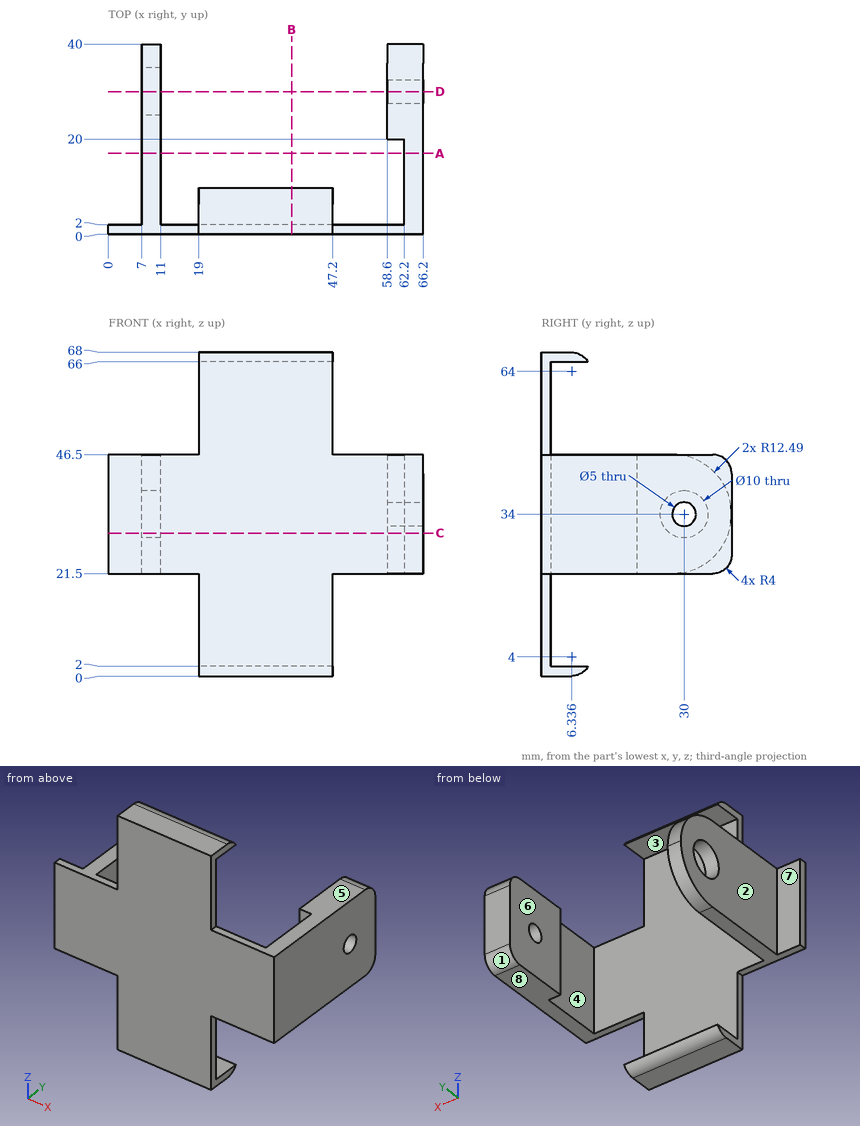
Source: three-view drawing plus pictorial views. Frame: mm from the lowest corner of the part. A direction names the side the tool comes from. Give positions to 0.01 mm unless a question says otherwise; leave off trailing zeros. Order: outer loops, then holes, each group sorted by start corner. A loop starts at its lowest first (then second) coordinate and runs counter-clockwise, first axis right, second up. Notation, with made-up numbers: (83.5, 3.25) - (141.5, 3.25) arc R21 cw to (141.5, 38.25) - close; hole circle Ø7 at (-28, 3). An arc over 180 degrees is marked (long way). Put each result on its own line as item: value.
Item 1: Draft query along Z for the marked faces 1, 2 and 3. Return one class per face: +Z half, -Z half, draft (parallel to the pull), parting line (faces both ways), or undercut.
Found:
face 1: -Z half
face 2: draft
face 3: undercut
Item 2: Section query C-C, the plane z = 30. Return loops of the section in (x, y), then the cut area to 3 significant figures.
Found:
outline: (0, 0) - (66.2, 0) - (66.2, 40) - (58.6, 40) - (58.6, 20) - (62.2, 20) - (62.2, 2) - (11, 2) - (11, 27) - (7, 27) - (7, 2) - (0, 2) - close; (7, 33) - (11, 33) - (11, 39.35) - (7, 39.35) - close
area: 482 mm^2
Item 3: Section query B-B, the plane x = 38.5. Return loops of the section in (y, z), then the cut area to 3 significant figures.
Found:
outline: (0, 0) - (6.34, 0) arc R4 ccw to (9.8, 2) - (2, 2) - (2, 66) - (9.8, 66) arc R4 ccw to (6.34, 68) - (0, 68) - close
area: 163 mm^2
Item 4: Section query A-A, the plane y = 17. Return loops of the section in (x, z), then the cut area to 3 significant figures.
Found:
outline: (7, 21.5) - (11, 21.5) - (11, 46.5) - (7, 46.5) - close; (62.2, 21.5) - (66.2, 21.5) - (66.2, 46.5) - (62.2, 46.5) - close
area: 200 mm^2
Item 5: Ray query, L1, parallel to Y at x = 61.25, z = 34; L2, parallel to Y at x = 8.2, z = 34; L3, parallel to X at y = 33, z = 42. Return the intervals inside material, ascending. Write a range as from..to.
Found:
L1: y = 0..2, 20..27.5, 32.5..40
L2: y = 0..25, 35..40
L3: x = 7..11, 58.6..66.2
Item 6: Section query D-D, the plane y = 30. Return loops of the section in (x, z), then the cut area to 3 significant figures.
Found:
outline: (7, 21.75) - (11, 21.75) - (11, 29) - (7, 29) - close; (7, 39) - (11, 39) - (11, 46.25) - (7, 46.25) - close; (58.6, 21.5) - (66.2, 21.5) - (66.2, 31.5) - (58.6, 31.5) - close; (58.6, 36.5) - (66.2, 36.5) - (66.2, 46.5) - (58.6, 46.5) - close
area: 210 mm^2
Item 7: Access query for the marked faces 4, 5, 6, 7 and 8. Directions: +Z, -Z, +X, -X, +Y, -Y. A direction counts if a zero-diameter tool reaches every point of the face in a straight line with its end or side. Return the directions, or none.
Found:
face 4: +Z, -Z
face 5: +Z, +X, +Y, -Y
face 6: +Z, -Z, +Y
face 7: +Z, -Z, -X, +Y
face 8: -Z, +X, +Y, -Y
Item 8: Contact query for flat-ended pins moving along their axis: pin 1 (15 mm diameter, centred on x = 53.5, y = 25.5, fed in from -Z); pin 2 (3 mm diameter, centred on x = 11.5, y = 33, fed in from -Z); pin 3 (8 mm diameter, centred on x = 7, z = 49.5, fed in from +Y). Output: stop coordinate, or through.
Found:
pin 1: stops at z = 21.5
pin 2: stops at z = 22.18
pin 3: stops at y = 32.41
